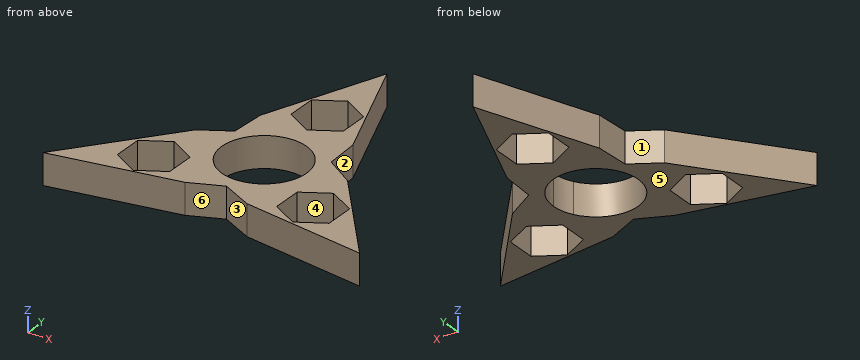
from build123d import *

# Parameters (mm, degrees)
F1_DEPTH = 8


# Not quite as in the source:
# - ends of sketch curves that miss each other by under 0.0002 mm in the source are joined


with BuildPart() as f1:
    # F0 (on Top) → F1 (new body)
    with BuildSketch(Plane.XY):
        Polygon((8.0340162625, -18.397915233), (40.4422496394, -23.3490666912), (19.9500470696, 2.2415004228), (12.4201863904, 7.1707647293), (11.9161368405, 16.1565585761), (0, 46.6985489201), (-11.9161368405, 16.1565585761), (-12.4201318249, 7.170681376), (-19.702678316, 2.9058864326), (-40.8897429157, -23.8067811423), (-8.2744899158, -17.8816622036), (0, -14.3414903669), align=None)
        Polygon((-20.4809666485, -4.0247617542), (-13.725968499, -7.9247617542), (-13.725968499, -15.7247617542), (-20.4809666485, -19.6247617542), (-27.2359647981, -15.7247617542), (-27.2359647981, -7.9247617542), align=None, mode=Mode.SUBTRACT)
        Polygon((13.9923272284, -15.8783317751), (13.9923272284, -8.0783317751), (20.7473253779, -4.1783317751), (27.5023235274, -8.0783317751), (27.5023235274, -15.8783317751), (20.7473253779, -19.7783317751), align=None, mode=Mode.SUBTRACT)
        with BuildLine():
            ThreePointArc((-9.4396629017, -5.4500242478), (-2.8211411141, 10.5285878832), (10.9, 0))
            ThreePointArc((10.9, 0), (10.5285987532, -2.8211005467), (9.4397049001, -5.4499515043))
            ThreePointArc((9.4397049001, -5.4499515043), (4.19985e-05, -10.8999999999), (-9.4396629017, -5.4500242478))
        make_face(mode=Mode.SUBTRACT)
        Polygon((6.7549981495, 27.9), (6.7549981495, 20.1), (0, 16.2), (-6.7549981495, 20.1), (-6.7549981495, 27.9), (0, 31.8), align=None, mode=Mode.SUBTRACT)
    extrude(amount=F1_DEPTH)


solid = f1.part
Work out the finished part from the listing and answer in its coordinate system (mm). Face numbers are marked on the shaded views. A direction names the side the tool comes from. Give positions to 0.01 mm unless a question says otherwise; leave off trailing zeros. Loops run counter-clockwise (first coordinate to the right, second up) from the corner with the lowest first, then second, coordinate; pieces in that order, holes last. Notation, with made-up numbers: (-39.75, -21.75) - (16.25, -21.75) arc R20 cw to (16.25, -6.75) - close; hole circle Ø3 at (38.5, 27). An arc over 180 degrees is marked (long way). Answer in a Markdown table with one row per item. Add a question column.
Q1. The part is cut by section D-D (x = -25). Determine the outline of the cut face in (y, z), and give its area (3 significant figures).
Q2. Consider line 1 along X through (y, z) = (18, 1.75); line 2 along X through (y, z) = (23.5, 4.75) (3 decimals); line 3 along X through (y, z) = (43.5, 1.5). Determine where each line is inside the solid, lowest interval first.
Q3. Each of these flat-tipped pins is pushed along its axis until it touches: P1, Ø1, axis at y = -16.5, z = 1, coming from the -X side; P2, Ø3, axis at x = -13.5, z = 4.5, coming from the -Y side; P3, Ø1, axis at x = -7, z = 6, coming from the -Y side. Where does it stop, or does it pass through?
Q4. Determine the mould class of the marked faces 1, 2 and 3 for opening direction X: released by +X, released by -X, zero draft, split by the parting line, or undercut.
Q5. The part is cut by section C-C (y = -10). Determine the outline of the cut face in (x, z), and give its area (3 significant figures).
Q6. The part is cut by section A-A (z = 5). State how many separate pieces and enclosed holes the cut face has, and give its area (3 significant figures).
Q7. A tool of negligible diameter and unlimited length cuts with its end or side. For the marked faces 4, 5 and 6, from which of +Z, -Z, +X, -X, +Y, -Y can it reach the whole face along a straight path? Write none if from no direction.
Q8. The part is cut by section B-B (x = 5). Determine the outline of the cut face in (y, z).
Solution:
| question | item | result |
|---|---|---|
| 1 | outline | (-20.92, 0) - (-17.02, 0) - (-17.02, 8) - (-20.92, 8) - close; (-6.63, 0) - (-3.77, 0) - (-3.77, 8) - (-6.63, 8) - close |
| 1 | area | 54.1 mm² |
| 2 | line 1 | x = -11.2 to -3.12, 3.12 to 11.2 |
| 2 | line 2 | x = -9.051 to -6.755, 6.755 to 9.051 |
| 2 | line 3 | x = -1.25 to 1.25 |
| 3 | P1 | stops at x = -35.49 |
| 3 | P2 | stops at y = -19.1 |
| 3 | P3 | stops at y = -17.55 |
| 4 | face 1 | released by -X |
| 4 | face 2 | released by +X |
| 4 | face 3 | undercut |
| 5 | outline | (-29.94, 0) - (-27.24, 0) - (-27.24, 8) - (-29.94, 8) - close; (-13.73, 0) - (-4.34, 0) - (-4.34, 8) - (-13.73, 8) - close; (4.34, 0) - (13.99, 0) - (13.99, 8) - (4.34, 8) - close; (27.5, 0) - (29.75, 0) - (29.75, 8) - (27.5, 8) - close |
| 5 | area | 192 mm² |
| 6 | separate pieces | 1 |
| 6 | enclosed holes | 4 |
| 6 | area | 1,170 mm² |
| 7 | face 4 | +Z, -Z |
| 7 | face 5 | -Z, +X, -X, +Y, -Y |
| 7 | face 6 | +Z, -Z, -Y |
| 8 | outline | (-16.87, 0) - (-9.69, 0) - (-9.69, 8) - (-16.87, 8) - close; (9.69, 0) - (19.09, 0) - (19.09, 8) - (9.69, 8) - close; (28.91, 0) - (33.88, 0) - (33.88, 8) - (28.91, 8) - close |
